```python
from build123d import *

# Parameters (mm, degrees)
F0_W     = 1060
F0_H     = 700
F1_DEPTH = 150
F2_SIZE  = 100
F3_W     = 920
F3_H     = 530
F4_DEPTH = 25


with BuildPart() as f1:
    # F0 (on Front) → F1 (new body)
    with BuildSketch(Plane.XZ):
        with Locations((530, 350)):
            Rectangle(F0_W, F0_H)
    extrude(amount=F1_DEPTH)

    # F2
    f2_edges = [f1.edges().sort_by_distance(p)[0] for p in [
        (1060, 0, 350),
        (530, 0, 700),
        (0, 0, 350),
        (530, 0, 0),
    ]]
    chamfer(f2_edges, length=F2_SIZE)

    # F3 (on face) → F4 (cut)
    with BuildSketch(Plane.XZ.offset(150)):
        with Locations((530, 385)):
            Rectangle(F3_W, F3_H)
    extrude(amount=-F4_DEPTH, mode=Mode.SUBTRACT)


solid = f1.part
```
The model under review builds one solid part; all positions refer to its coordinate system, in mm. A direction names the side the tool comes from. Coordinates: 2 decimals unless noted, no trailing zeros. Write each loop counter-clockwise with the first axis right and the second up, starting at its lowest first coordinate (ties: lowest second). Pieces come first, ordered by that corner, then holes. Notation, with made-up numbers: (80, 1.5) - (89, 1.5) arc R34 cw to (89, 32.5) - close; hole circle Ø6 at (4.25, 27). An arc over 180 degrees is marked (long way). Answer in a Markdown table with one row per item. Add a question column.
Q1. Consider section C-C on y = -13. Give the boundary of the cut face in (x, z), then the cut area to 3 significant figures.
Q2. Consider section A-A on z = 535. Give the boundary of the cut face in (x, y), then the cut area to 3 significant figures.
Q3. To check wall thickness, follow line 1 along X through (y, z) = (-141, 400); line 2 along Y through (x, z) = (233, 412.5); line 3 along X through (y, z) = (-51.5, 148.5). State the ranges of each line that lie inside material, in increasing order. Write a range as from..to.
Q4. Draft analysis for pull direction X (two halves, no side actions). For faces 1 (the face through (523, -150, 44)), 2 (the face through (1009, -49, 345)), 3 (the face through (70, -138, 381)), 4 (the face through (990, -138, 381)), state which applies: +X half, -X half, draft (parallel to the pull), parting line (faces both ways), or undercut.
Q5. For faces 5 (the face through (524, -125, 389)), 6 (the face through (524, 0, 354)), list the 3-axis set-ups (+Z, -Z, +X, -X, +Y, -Y) from which the entire face can be reached by the end or side of a thin tool; tool diameter is ignored.
Q6. Consider section B-B on x = 819. Give the boundary of the cut face in (y, z), then the cut area to 4 significant figures.
Q7. Clearance check with flat-ended pins moving along their axes: pin 1 (2 mm diameter, centred on y = -27, z = 534.5, fed in from -X); pin 2 (1 mm diameter, centred on x = 602, y = -92, fed in from -Z); pin 3 (8 mm diameter, centred on x = 563.5, y = -90, fed in from +Z). State where each tip first meets the part, or that it passes through.
Q8. Consider section D-D on z = 87.5. Give the boundary of the cut face in (x, y).
Answers below:
| question | item | result |
|---|---|---|
| 1 | outline | (87, 87) - (973, 87) - (973, 613) - (87, 613) - close |
| 1 | area | 466,000 mm² |
| 2 | outline | (0, -150) - (70, -150) - (70, -125) - (990, -125) - (990, -150) - (1060, -150) - (1060, -100) - (960, 0) - (100, 0) - (0, -100) - close |
| 2 | area | 126,000 mm² |
| 3 | line 1 | 0..70, 990..1060 |
| 3 | line 2 | -125..0 |
| 3 | line 3 | 48.5..1011.5 |
| 4 | face 1 | draft |
| 4 | face 2 | +X half |
| 4 | face 3 | undercut |
| 4 | face 4 | undercut |
| 5 | face 5 | -Y |
| 5 | face 6 | +Z, -Z, +X, -X, +Y |
| 6 | outline | (-150, 0) - (-100, 0) - (0, 100) - (0, 600) - (-100, 700) - (-150, 700) - (-150, 650) - (-125, 650) - (-125, 120) - (-150, 120) - close |
| 6 | area | 81,750 mm² |
| 7 | pin 1 | x = 72 |
| 7 | pin 2 | z = 7.5 |
| 7 | pin 3 | z = 694 |
| 8 | outline | (0, -150) - (1060, -150) - (1060, -100) - (972.5, -12.5) - (87.5, -12.5) - (0, -100) - close |
